Part model, mm, in its own coordinate system. Give positions to 0.01 mm unless a question says otherwise; leave off trailing zeros. Loops run counter-clockwise (first coordinate to the right, second up) from the corner with the lowest first, then second, coordinate; pieces in that order, holes last. Notation, with made-up numbers: M -14,80 L -2,80 A24 ccw -2,93 Z; hole C 56,70.25 d1. An arc over 180 degrees is marked long. Answer in a Markdown table with one row per item.
from build123d import *

# Parameters (mm, degrees)
SKETCH1_R           = 1.75
BOSS_EXTRUDE1_DEPTH = 6.35
SKETCH2_R           = 1.75
CUT_EXTRUDE1_DEPTH  = 10


with BuildPart() as part:
    # Sketch1 → Boss-Extrude1 (new body)
    with BuildSketch(Plane.XY):
        with BuildLine():
            Line((0, 1), (0, 109))
            ThreePointArc((0, 109), (0.292893219, 109.707106781), (1, 110))
            Line((1, 110), (9, 110))
            ThreePointArc((9, 110), (9.707106781, 109.707106781), (10, 109))
            Line((10, 109), (10, 1))
            ThreePointArc((10, 1), (9.707106781, 0.292893219), (9, 0))
            Line((9, 0), (1, 0))
            ThreePointArc((1, 0), (0.292893219, 0.292893219), (0, 1))
        make_face()
        with Locations((5, 105)):
            Circle(SKETCH1_R, mode=Mode.SUBTRACT)
        with Locations((5, 5)):
            Circle(SKETCH1_R, mode=Mode.SUBTRACT)
    extrude(amount=BOSS_EXTRUDE1_DEPTH)

    # Sketch2 → Cut-Extrude1 (cut)
    with BuildSketch(Plane.XY.offset(6.35)):
        with Locations((5, 25)):
            Circle(SKETCH2_R)
    extrude(amount=-CUT_EXTRUDE1_DEPTH, mode=Mode.SUBTRACT)


solid = part.part
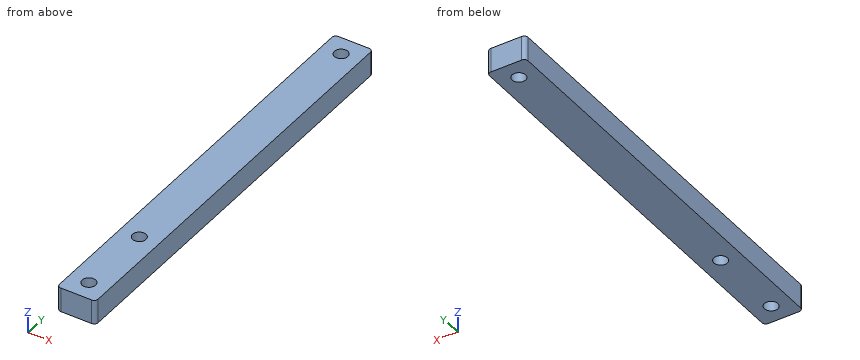
(1) Pin check, flat tip, straight feed: pin 1 Ø1.5 at (x, y) = (2, 93) entering from -Z. Stop position of the tip, or through.
Recorded:
| item | result |
|---|---|
| pin 1 | stops at z = 0 |
(2) Saw through at A-A (z = 2). Write the cut outline in (x, y), plus the area to 3 significant figures.
Recorded:
| item | result |
|---|---|
| outline | M 0,1 A1 ccw 1,0 L 9,0 A1 ccw 10,1 L 10,109 A1 ccw 9,110 L 1,110 A1 ccw 0,109 Z; hole C 5,5 d3.5; hole C 5,25 d3.5; hole C 5,105 d3.5 |
| area | 1,070 mm^2 |
(3) Saw through at C-C (x = 5). Write the cut outline in (y, z).
Recorded:
| item | result |
|---|---|
| outline | M 0,0 L 3.25,0 L 3.25,6.35 L 0,6.35 Z; M 6.75,0 L 23.25,0 L 23.25,6.35 L 6.75,6.35 Z; M 26.75,0 L 103.25,0 L 103.25,6.35 L 26.75,6.35 Z; M 106.75,0 L 110,0 L 110,6.35 L 106.75,6.35 Z |
(4) Saw through at B-B (y = 105). Write the cut outline in (x, z), plus the area to 3 significant figures.
Recorded:
| item | result |
|---|---|
| outline | M 0,0 L 3.25,0 L 3.25,6.35 L 0,6.35 Z; M 6.75,0 L 10,0 L 10,6.35 L 6.75,6.35 Z |
| area | 41.3 mm^2 |
(5) Drill centre lines: line 1 along Y through (x, z) = (5, 3.25); line 2 along Y through (x, z) = (5.75, 2.5); line 3 along X through (y, z) = (105, 1.5). Where is each one in solid material? Low to high.
Recorded:
| item | result |
|---|---|
| line 1 | y = 0 to 3.25, 6.75 to 23.25, 26.75 to 103.25, 106.75 to 110 |
| line 2 | y = 0 to 3.42, 6.58 to 23.42, 26.58 to 103.42, 106.58 to 110 |
| line 3 | x = 0 to 3.25, 6.75 to 10 |
